Model file for the job. Use its own axes, mm. A direction names the side the tool comes from. Give positions to 0.01 mm unless a question says otherwise; leave off trailing zeros. Write each loop counter-clockwise with the first axis right and the second up, starting at its lowest first coordinate (ties: lowest second). Pieces come first, ordered by that corner, then holes.
```python
from build123d import *

# Parameters (mm, degrees)
SKETCH1_R           = 5.05
BOSS_EXTRUDE1_DEPTH = 5
BOSS_EXTRUDE2_START = 5
BOSS_EXTRUDE2_DEPTH = 5
BOSS_EXTRUDE4_DEPTH = 2
CUT_EXTRUDE1_START  = -3
SKETCH6_R           = 9.5
SKETCH6_R_2         = 5.05
CUT_EXTRUDE1_DEPTH  = 3
SKETCH7_R           = 2.5
CUT_EXTRUDE2_DEPTH  = 74.87151007
SKETCH8_R           = 4
BOSS_EXTRUDE5_DEPTH = 3
CUT_EXTRUDE3_DEPTH  = 3
SKETCH10_W          = 8.596273884
SKETCH10_H          = 2
CUT_REVOLVE1_ANGLE  = 180
SKETCH12_R          = 2


with BuildPart() as part:
    # Sketch1 → Boss-Extrude1 (new body)
    with BuildSketch(Plane.XY):
        with BuildLine():
            Line((-52, 0), (52, 0))
            ThreePointArc((52, 0), (0, -52), (-52, 0))
        make_face()
        with Locations((-20, -20)):
            Circle(SKETCH1_R, mode=Mode.SUBTRACT)
    extrude(amount=-BOSS_EXTRUDE1_DEPTH)

    # Sketch2 → Boss-Extrude2 (add)
    with BuildSketch(Plane.XY.offset(BOSS_EXTRUDE2_START)):
        with BuildLine():
            Line((52, 0), (-52, 0))
            ThreePointArc((-52, 0), (0, -52), (52, 0))
        make_face()
        with BuildLine():
            Line((49.959983987, -2), (-49.959983987, -2))
            ThreePointArc((-49.959983987, -2), (0, -50), (49.959983987, -2))
        make_face(mode=Mode.SUBTRACT)
    extrude(amount=-BOSS_EXTRUDE2_DEPTH)

    # Sketch5 → Boss-Extrude4 (add)
    with BuildSketch(Plane(origin=(0, 0, -5), x_dir=(-1, 0, 0), z_dir=(0, 0, -1))):
        with BuildLine():
            ThreePointArc((-49.323463146, -16.468029126), (-45.033320997, -26), (-38.923463146, -34.481357524))
            Line((-38.923463146, -34.481357524), (-37.426406871, -33.155151466))
            ThreePointArc((-37.426406871, -33.155151466), (-43.301270189, -25), (-47.426406871, -15.83464339))
            Line((-47.426406871, -15.83464339), (-49.323463146, -16.468029126))
        make_face()
        with BuildLine():
            Line((10.4, -50.94938665), (10, -48.989794856))
            ThreePointArc((10, -48.989794856), (0, -50), (-10, -48.989794856))
            Line((-10, -48.989794856), (-10.4, -50.94938665))
            ThreePointArc((-10.4, -50.94938665), (0, -52), (10.4, -50.94938665))
        make_face()
        with BuildLine():
            Line((37.426406871, -33.155151466), (38.923463146, -34.481357524))
            ThreePointArc((38.923463146, -34.481357524), (45.033320997, -26), (49.323463146, -16.468029126))
            Line((49.323463146, -16.468029126), (47.426406871, -15.83464339))
            ThreePointArc((47.426406871, -15.83464339), (43.301270189, -25), (37.426406871, -33.155151466))
        make_face()
    extrude(amount=BOSS_EXTRUDE4_DEPTH)

    # Sketch6 → Cut-Extrude1 (cut)
    with BuildSketch(Plane(origin=(0, 0, -5), x_dir=(-1, 0, 0), z_dir=(0, 0, -1)).offset(CUT_EXTRUDE1_START)):
        with Locations((0, -20)):
            Circle(SKETCH6_R)
        with Locations(Location((20, -20, 0), (0, 0, 180))):
            Circle(SKETCH6_R_2)
    extrude(amount=CUT_EXTRUDE1_DEPTH, mode=Mode.SUBTRACT)

    # Sketch7 → Cut-Extrude2 (cut, through all)
    with BuildSketch(Plane(origin=(0, 0, -2), x_dir=(-1, 0, 0), z_dir=(0, 0, -1))):
        with Locations((0, -20)):
            Circle(SKETCH7_R)
    extrude(amount=-CUT_EXTRUDE2_DEPTH, mode=Mode.SUBTRACT)

    # Sketch8 → Boss-Extrude5 (add)
    with BuildSketch(Plane(origin=(0, 0, -5), x_dir=(-1, 0, 0), z_dir=(0, 0, -1))):
        with Locations(Location((-20, -20, 0), (0, 0, 180))):
            Circle(SKETCH8_R)
    extrude(amount=BOSS_EXTRUDE5_DEPTH)

    # Sketch9 → Cut-Extrude3 (cut)
    # profile 1 of 2: a face of its own
    with BuildSketch(Plane.XY.offset(5)):
        with BuildLine():
            Line((50.990195136, -1), (-50.990195136, -1))
            ThreePointArc((-50.990195136, -1), (0, -51), (50.990195136, -1))
        make_face()
        with BuildLine():
            ThreePointArc((49.959983987, -2), (0, -50), (-49.959983987, -2))
            Line((-49.959983987, -2), (49.959983987, -2))
        make_face(mode=Mode.SUBTRACT)
    # profile 2 of 2: a face of its own
    with BuildSketch(Plane.XY.offset(5)):
        with BuildLine():
            Line((-49.959983987, -2), (49.959983987, -2))
            ThreePointArc((49.959983987, -2), (0, -50), (-49.959983987, -2))
        make_face()
    extrude(amount=-CUT_EXTRUDE3_DEPTH, mode=Mode.SUBTRACT)

    # Sketch10 → Cut-Revolve1 (revolve, cut)
    with BuildSketch(Plane(origin=(0, 0, 0), x_dir=(1, 0, 0), z_dir=(0, 1, 0))):
        with Locations((54.298136942, 2)):
            Rectangle(SKETCH10_W, SKETCH10_H)
    revolve(axis=Axis((0, 0, -7.000025), (0, 0, -1)), revolution_arc=CUT_REVOLVE1_ANGLE, mode=Mode.SUBTRACT)

    # Sketch12 → Cut-Revolve2 (revolve, cut)
    with BuildSketch(Plane(origin=(0, -20, 0), x_dir=(1, 0, 0), z_dir=(0, 1, 0)), mode=Mode.PRIVATE) as cut_revolve2_sk:
        with Locations((-12, 5)):
            Circle(SKETCH12_R)
    revolve(cut_revolve2_sk.sketch.rotate(Axis((-20, -20, -5), (0, 0, 1)), 180), axis=Axis((-20, -20, -5), (0, 0, 1)), mode=Mode.SUBTRACT)


solid = part.part
```
1. Pin check, flat tips, straight feed: P1, Ø13, axis at x = -45.5, y = -26, coming from the -Z side; P2, Ø2, axis at x = 22, z = 1.5, coming from the -Y side; P3, Ø9.5, axis at x = 1.5, y = -18.5, coming from the -Z side. Stop position of each tip, or through.
Calculated:
P1: stops at z = -7
P2: stops at y = -47.57
P3: stops at z = -2
2. Slice it at C-C, the plane x = -40.5. Write the cut outline in (y, z), and give its area (3 significant figures).
Calculated:
outline: (-32.62, -7) - (-29.32, -7) - (-29.32, -5) - (0, -5) - (0, 5) - (-1, 5) - (-1, 2) - (-2, 2) - (-2, 0) - (-29.32, 0) - (-29.32, 2) - (-31, 2) - (-31, 5) - (-32.62, 5) - (-32.62, -1) - (-29.32, -1) - (-29.32, -3) - (-32.62, -3) - close
area: 182 mm2
3. Pull direction Y, two halves, no side cores. Call faces 6 (the cylindrical face through (1.099, -49.988, -2.014)), 7 (the cylindrical face through (-1.34, -17.89, -1.01)), 8 (the flat face through (1, 0, 0)): +Y half, -Y half, draft (parallel to the pull), parting line (faces both ways), or undercut.
Calculated:
face 6: -Y half
face 7: undercut
face 8: +Y half
4. Slice it at D-D, the plane y = -20. State how many separate pieces and enclosed holes the cut face has, and give its area (3 significant figures).
Calculated:
separate pieces: 3
enclosed holes: 0
area: 389 mm2
5. Slice it at B-B, the plane y = -37.5. Write the cut outline in (x, z), and give its area (3 significant figures).
Calculated:
outline: (-36.02, -5) - (36.02, -5) - (36.02, -3) - (33.07, -3) - (33.07, -1) - (36.02, -1) - (36.02, 5) - (34.57, 5) - (34.57, 2) - (33.07, 2) - (33.07, 0) - (-33.07, 0) - (-33.07, 2) - (-34.57, 2) - (-34.57, 5) - (-36.02, 5) - (-36.02, -1) - (-33.07, -1) - (-33.07, -3) - (-36.02, -3) - close
area: 369 mm2
6. Which spindle directions (+Z, -Z, +X, -X, +Y, -Y) get a long thin tool onto all of the face, cutting with end or side? Do faces 1 (the flat face through (-48.388, -16.156, -5.986)), 2 (the cylindrical face through (0, -50, -6)), 3 (the flat face through (1, -1, 4)), 4 (the flat face through (-2, -22, -2)), 5 (the flat face through (-44, -26, -7)). Say none if no direction does.
Calculated:
face 1: -Z, -X, +Y
face 2: -Z, +Y
face 3: +Z
face 4: -Z
face 5: -Z, -X, +Y, -Y
7. Probe probe 1 along Y at (x, z) = (0, -4.15); probe 2 along Z at (x, y) = (26, -45); probe 3 along Y at (x, z) = (0, -1.15). List the from-to ranges inside material, lowest first.
Calculated:
probe 1: y = -52 to -29.5, -10.5 to 0
probe 2: z = -5 to -3, -1 to 5
probe 3: y = -50 to -22.5, -17.5 to 0
8. Slice it at A-A, the plane x = 0. Write the cut outline in (y, z).
Calculated:
outline: (-52, -7) - (-50, -7) - (-50, -5) - (-29.5, -5) - (-29.5, -2) - (-22.5, -2) - (-22.5, 0) - (-50, 0) - (-50, 2) - (-51, 2) - (-51, 5) - (-52, 5) - (-52, -1) - (-50, -1) - (-50, -3) - (-52, -3) - close; (-17.5, -2) - (-10.5, -2) - (-10.5, -5) - (0, -5) - (0, 5) - (-1, 5) - (-1, 2) - (-2, 2) - (-2, 0) - (-17.5, 0) - close
